Answer from the drawing. Dimensions are ordinates in mm from the lowest x, y and z of the part. A direction names the side the tool comes from. Coordinates: 2 decimals unless noted, no trailing zeros. Loops run counter-clockwise (first coordinate to the right, second up) from the corner with the lowest first, then second, coordinate; pieces in that order, holes last. Notation, with made-up numbers: (-20.75, 76) - (15.25, 76) arc R23 cw to (15.25, 105) - close; hole circle Ø2 at (-33.75, 88). An arc over 180 degrees is marked (long way). Use one line per item in the form item = value. Start each with the question number.
1) A cutting plane is placed at D-D (x = 5.5). Give the vertices of the cut face in (y, z).
2) Each of these flat-tipped pins is pushed along its axis until it touches: P1, Ø5.5, axis at y = 5, z = 17, coming from the +X side; P2, Ø1.5, axis at y = 5, z = 1.5, coming from the +X side; P3, Ø7.5, axis at x = 27, z = 7, coming from the -Y side; P4, Ø5, axis at x = 6, y = 40, coming from the -Z side. Where does it stop, or does it pass through?
3) A cutting plane is placed at C-C (y = 13). Give the vertices of the cut face in (x, z), and give its area (3 significant figures).
4) The mould has two halves that part along Y. Classify the marked faces 1, 2 and 3: released by +Y, released by -Y, zero draft, split by the parting line, or undercut.
5) A cutting plane is placed at A-A (z = 3). Give the vertices of the cut face in (x, y) (1 decimal).
6) Consider line 1 (Z direction, x = 23, y = 3.5); line 2 (X direction, y = 26, z = 11.5) (1 decimal); line 3 (Z direction, x = 45.5, y = 10). Determine where each line is inside the solid, lowest interval first.
7) Which of the six approach directions +Z, -Z, +X, -X, +Y, -Y give full straight-line access (tool end or side, diameter ignored) to the marked faces 4, 5, 6 and 7?
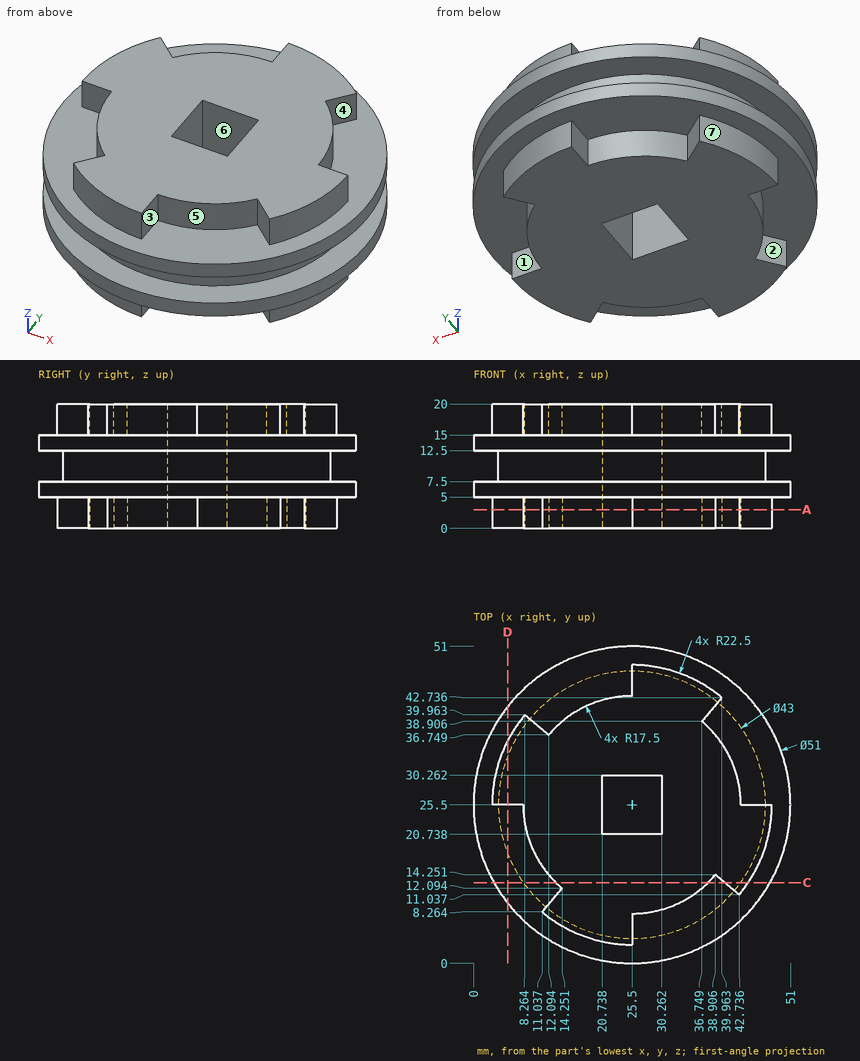
Found:
q1.outline = (9.68, 5) - (25.5, 5) - (25.5, 0) - (35.81, 0) - (35.81, 5) - (41.32, 5) - (41.32, 7.5) - (33.39, 7.5) - (33.39, 12.5) - (41.32, 12.5) - (41.32, 15) - (35.81, 15) - (35.81, 20) - (25.5, 20) - (25.5, 15) - (9.68, 15) - (9.68, 12.5) - (17.61, 12.5) - (17.61, 7.5) - (9.68, 7.5) - close
q2.P1 = 42.93
q2.P2 = 25.5
q2.P3 = 0
q2.P4 = 0
q3.outline = (3.27, 5) - (13.25, 5) - (13.25, 0) - (37.75, 0) - (37.75, 5) - (40.4, 5) - (40.4, 0) - (44.21, 0) - (44.21, 5) - (47.73, 5) - (47.73, 7.5) - (42.99, 7.5) - (42.99, 12.5) - (47.73, 12.5) - (47.73, 15) - (44.21, 15) - (44.21, 20) - (40.4, 20) - (40.4, 15) - (37.75, 15) - (37.75, 20) - (13.25, 20) - (13.25, 15) - (3.27, 15) - (3.27, 12.5) - (8.01, 12.5) - (8.01, 7.5) - (3.27, 7.5) - close
q3.area = 680 mm^2
q4.face_1 = released by +Y
q4.face_2 = undercut
q4.face_3 = zero draft
q5.outline = (3, 25.5) - (8, 25.5) arc R17.5 ccw to (14.3, 12.1) - (11, 8.3) arc R22.5 ccw to (25.5, 3) - (25.5, 8) arc R17.5 ccw to (38.9, 14.3) - (42.7, 11) arc R22.5 ccw to (48, 25.5) - (43, 25.5) arc R17.5 ccw to (36.7, 38.9) - (40, 42.7) arc R22.5 ccw to (25.5, 48) - (25.5, 43) arc R17.5 ccw to (12.1, 36.7) - (8.3, 40) arc R22.5 ccw to start; hole (20.7, 20.7) - (30.3, 20.7) - (30.3, 30.3) - (20.7, 30.3) - close
q6.line_1 = 0 to 7.5, 12.5 to 20
q6.line_2 = 4 to 20.7, 30.3 to 47
q6.line_3 = 5 to 7.5, 12.5 to 15
q7.face_4 = +Z, +X
q7.face_5 = +Z, -Y
q7.face_6 = +Z, -Z
q7.face_7 = -Z, -X, +Y
